Read the model definition and answer for the solid it produces. Units are mm, in the model's axes. A direction names the side the tool comes from. Give positions to 0.01 mm unless a question says otherwise; leave off trailing zeros. Write each loop counter-clockwise with the first axis right and the second up, starting at its lowest first coordinate (ties: lowest second). Pieces come first, ordered by that corner, then holes.
```python
from build123d import *

# Parameters (mm, degrees)
BOSS_EXTRUDE1_DEPTH = 5
CUT_EXTRUDE1_DEPTH  = 1
SKETCH3_R           = 3.5
BOSS_EXTRUDE2_DEPTH = 2
CUT_EXTRUDE2_DEPTH  = 5


with BuildPart() as part:
    # Sketch1 → Boss-Extrude1 (new body)
    with BuildSketch(Plane(origin=(0, 0, 0), x_dir=(1, 0, 0), z_dir=(0, 1, 0))):
        with BuildLine():
            Line((-45, -25), (45, -25))
            ThreePointArc((45, -25), (48.535533906, -23.535533906), (50, -20))
            Line((50, -20), (50, 20))
            ThreePointArc((50, 20), (48.535533906, 23.535533906), (45, 25))
            Line((45, 25), (-45, 25))
            ThreePointArc((-45, 25), (-48.535533906, 23.535533906), (-50, 20))
            Line((-50, 20), (-50, -20))
            ThreePointArc((-50, -20), (-48.535533906, -23.535533906), (-45, -25))
        make_face()
    extrude(amount=BOSS_EXTRUDE1_DEPTH)

    # Sketch2 → Cut-Extrude1 (cut)
    with BuildSketch(Plane(origin=(0, 0, 0), x_dir=(-1, 0, 0), z_dir=(0, -1, 0))):
        with BuildLine():
            Line((-43.707715382, -20), (-30.707715382, -20))
            ThreePointArc((-30.707715382, -20), (-30.0006086, -19.707106781), (-29.707715382, -19))
            Line((-29.707715382, -19), (-29.707715382, -6))
            ThreePointArc((-29.707715382, -6), (-30.0006086, -5.292893219), (-30.707715382, -5))
            Line((-30.707715382, -5), (-43.707715382, -5))
            ThreePointArc((-43.707715382, -5), (-44.414822163, -5.292893219), (-44.707715382, -6))
            Line((-44.707715382, -6), (-44.707715382, -19))
            ThreePointArc((-44.707715382, -19), (-44.414822163, -19.707106781), (-43.707715382, -20))
        make_face()
    extrude(amount=-CUT_EXTRUDE1_DEPTH, mode=Mode.SUBTRACT)

    # Sketch3 → Boss-Extrude2 (add)
    with BuildSketch(Plane(origin=(0, 1, 0), x_dir=(-1, 0, 0), z_dir=(0, -1, 0))):
        with Locations(Location((-37.914895337, -8.755915312, 0), (0, 0, 270))):
            Circle(SKETCH3_R)
        with Locations(Location((-34.024612955, -14.842826033, 0), (0, 0, 270))):
            Circle(SKETCH3_R)
        with Locations(Location((-41.209446078, -15.261216115, 0), (0, 0, 181.801905024))):
            Circle(SKETCH3_R)
    extrude(amount=BOSS_EXTRUDE2_DEPTH)

    # Sketch4 → Cut-Extrude2 (cut)
    with BuildSketch(Plane.ZY.offset(50)):
        with BuildLine():
            Line((2, 1.770486386), (-2, 1.770486386))
            ThreePointArc((-2, 1.770486386), (-2.353553391, 1.916932996), (-2.5, 2.270486386))
            Line((-2.5, 2.270486386), (-2.5, 3.270486386))
            ThreePointArc((-2.5, 3.270486386), (-2.353553391, 3.624039777), (-2, 3.770486386))
            Line((-2, 3.770486386), (2, 3.770486386))
            ThreePointArc((2, 3.770486386), (2.353553391, 3.624039777), (2.5, 3.270486386))
            Line((2.5, 3.270486386), (2.5, 2.270486386))
            ThreePointArc((2.5, 2.270486386), (2.353553391, 1.916932996), (2, 1.770486386))
        make_face()
    extrude(amount=-CUT_EXTRUDE2_DEPTH, mode=Mode.SUBTRACT)


solid = part.part
```
Item 1: Which of the six approach directions +Z, -Z, +X, -X, +Y, -Y give full straight-line access (tool end or side, diameter ignored) to faces 1 (the flat face through (41, -1, 15)), 2 (the cylindrical face through (30.554, 0.014, 14.387)), 3 (the flat face through (-45, 3, 0))?
Result set:
face 1: +Z, -Z, +X, -X, -Y
face 2: -Y
face 3: -X
Item 2: Determine the mould class of faces 4 (the flat face through (-48, 3.77, 0)), 5 (the cylindrical face through (34.445, 0.014, 8.3)), 6 (the flat face through (37.3, 1, 12.4)) for opening direction Y: pulls with the +Y half, pulls with the -Y half, needs draft (parallel to the pull), parting line crosses it, or undercut.
Result set:
face 4: undercut
face 5: needs draft
face 6: pulls with the -Y half
Item 3: Section B-B (z = -3.5) is taken. Write down the section's boundary in (x, y), and give its area (3 significant figures).
Result set:
outline: (-50, 0) - (50, 0) - (50, 5) - (-50, 5) - close
area: 500 mm2
Item 4: Each of these flat-tipped pins is pushed along its axis until it touches: pin 1 Ø0.8 at (x, y) = (-48, 3) entering from +Z; pin 2 Ø16.5 at (x, z) = (34.5, 11) entering from -Y; pin 3 Ø2 at (x, z) = (-47.5, 0) entering from -Y; pin 4 Ø0.5 at (x, y) = (-47.5, 2.5) entering from -Z. Where does it stop, or does it pass through?
Result set:
pin 1: stops at z = 24.27
pin 2: stops at y = -1
pin 3: stops at y = 0
pin 4: stops at z = -24.47
Item 5: Find the intervals of material crossed by line 1 along Z through (x, y) = (34, 0.35); line 2 along Y through (x, z) = (45.5, -3); line 3 along X through (y, z) = (-0.1, 6), in increasing order.
Result set:
line 1: z = -25 to 5, 11.34 to 18.34, 20 to 25
line 2: y = 0 to 5
line 3: x = 35.76 to 40.07
Item 6: Section A-A (x = -33.5) is taken. Write down the section's boundary in (y, z).
Result set:
outline: (0, -25) - (5, -25) - (5, 25) - (0, 25) - close
